Source: CAD feature listing. Evaluate the final solid. Frame: model axes, mm. A direction names the side the tool comes from. Give positions to 0.01 mm unless a question says otherwise; leave off trailing zeros. Order: outer loops, then holes, each group sorted by start corner. A loop starts at its lowest first (then second) coordinate and runs counter-clockwise, first axis right, second up. Notation, with made-up numbers: M -30,-6 L 3,-6 A17 cw 3,13 Z; hole C 3.5,-21 d6. An arc over 180 degrees is marked long. Use CSV: the item, a comma, the result in double quotes. Start each with the question number.
Item 1: Pull-direction query (Z, two-part tool) for faces 3 (the face through (57.719, 0.805, -94.535)), 4 (the face through (59.9, 0.8, -78.5)), 5 (the face through (59.97, 0.78, -120.62)), 6 (the face through (29.81, 0.78, -196.55)); classes: +Z half, -Z half, draft (parallel to the pull), parting line (faces both ways), or undercut.
Item 2: Section query A-A on z = -56.67. Return loops of the section in (x, y).
Item 3: First-contact query: pin 1 (0.5 mm diameter, centred on x = 16.5, y = 1, fed in from -Z); pin 2 (2.5 mm diameter, centred on x = 43.45, z = -42.87, fed in from -Y). Flat tips, straight axial feed; report the tip coordinate or a pass-through.
Item 4: Section query B-B on x = 55.5. Return loops of the section in (y, z), and give its area (3 significant figures).
Item 5: Access query for faces 1 (the face through (6.493, 0.783, -108.844)), 2 (the face through (3.66, 0.78, -167.99)). Directions: +Z, -Z, +X, -X, +Y, -Y. A direction counts if a zero-diameter tool reaches every point of the face in a straight line with its end or side. Return the directions, or none.
Item 6: Section query C-C on y = 0.3. Count the separate pieces of the cut face and the enclosed holes in it, and give its area (3 significant figures).
Item 7: Ray query, probe 1 along X at (y, z) = (0.8, -56.67); probe 2 along X at (y, z) = (0.25, -71); probe 3 along X at (y, z) = (0.65, -185). Return the intervals inside material, ascending. Write a range as from..to.
from build123d import *

# Parameters (mm, degrees)
SKETCH1_R           = 1.388229101
SKETCH1_R_2         = 1.896979128
SKETCH1_R_3         = 2
SKETCH1_R_4         = 1.314910669
SKETCH1_R_5         = 1.483383261
SKETCH1_R_6         = 1.248623853
SKETCH1_R_7         = 1.255629307
SKETCH1_R_8         = 7
SKETCH1_R_9         = 1.53911217
BOSS_EXTRUDE1_DEPTH = 1.5875
SKETCH4_W           = 66.272407177
SKETCH4_H           = 27.800260981
CUT_EXTRUDE2_DEPTH  = 20
FILLET3_R           = 10
FILLET4_R           = 10
BOSS_EXTRUDE3_START = -1.5875
BOSS_EXTRUDE3_DEPTH = 1.5875
SKETCH7_R           = 7
CUT_EXTRUDE3_DEPTH  = 1.5875
SKETCH8_W           = 100.106183873
SKETCH8_H           = 60.21728362
CUT_EXTRUDE4_DEPTH  = 35
FILLET5_R           = 10


with BuildPart() as part:
    # Sketch1 → Boss-Extrude1 (new body)
    with BuildSketch(Plane(origin=(0, 0, 0), x_dir=(1, 0, 0), z_dir=(0, 1, 0))):
        with BuildLine():
            Line((42.32729629, 228.6), (10.454309325, 228.6))
            Line((10.454309325, 228.6), (0, 135.362739137))
            Line((0, 135.362739137), (0, 0))
            Line((0, 0), (24.327009544, 0))
            Line((24.327009544, 0), (50.8, 0))
            Line((50.8, 0), (50.8, 64.87909603))
            Line((50.8, 64.87909603), (50.8, 87.423477361))
            Line((50.8, 87.423477361), (50.8, 98.200996728))
            ThreePointArc((50.8, 98.200996728), (50.4, 101.000996728), (50.8, 103.800996728))
            Line((50.8, 103.800996728), (50.8, 104.488200565))
            Line((50.8, 104.488200565), (50.8, 120.619222808))
            Line((50.8, 120.619222808), (50.8, 135.362739137))
            Line((50.8, 135.362739137), (42.32729629, 228.6))
        make_face()
        with Locations(Location((6.335590122, 44.288799513, 0), (0, 0, 270))):
            Circle(SKETCH1_R, mode=Mode.SUBTRACT)
        with Locations(Location((16.545548495, 56.66670766, 0), (0, 0, 270))):
            Circle(SKETCH1_R_2, mode=Mode.SUBTRACT)
        with Locations(Location((32.542900948, 56.67, 0), (0, 0, 270))):
            Circle(SKETCH1_R_3, mode=Mode.SUBTRACT)
        with Locations(Location((4.659546827, 82.793173401, 0), (0, 0, 270))):
            Circle(SKETCH1_R_4, mode=Mode.SUBTRACT)
        with Locations(Location((16.254490953, 72.66670766, 0), (0, 0, 270))):
            Circle(SKETCH1_R_3, mode=Mode.SUBTRACT)
        with Locations(Location((32.251843406, 72.67, 0), (0, 0, 270))):
            Circle(SKETCH1_R_3, mode=Mode.SUBTRACT)
        with BuildLine():
            Line((34.925740903, 92.78493524), (9.492033273, 92.78493524))
            ThreePointArc((9.492033273, 92.78493524), (6.992033273, 95.28493524), (9.492033273, 97.78493524))
            Line((9.492033273, 97.78493524), (34.925740903, 97.78493524))
            ThreePointArc((34.925740903, 97.78493524), (36.693507856, 97.052702193), (37.425740903, 95.28493524))
            ThreePointArc((37.425740903, 95.28493524), (36.693507856, 93.517168287), (34.925740903, 92.78493524))
        make_face(mode=Mode.SUBTRACT)
        with BuildLine():
            Line((34.925740903, 105.90993524), (9.492033273, 105.90993524))
            ThreePointArc((9.492033273, 105.90993524), (6.492033273, 108.90993524), (9.492033273, 111.90993524))
            Line((9.492033273, 111.90993524), (34.925740903, 111.90993524))
            ThreePointArc((34.925740903, 111.90993524), (37.047061246, 111.031255584), (37.925740903, 108.90993524))
            ThreePointArc((37.925740903, 108.90993524), (37.047061246, 106.788614896), (34.925740903, 105.90993524))
        make_face(mode=Mode.SUBTRACT)
        with Locations(Location((43.447673368, 42.868436544, 0), (0, 0, 270))):
            Circle(SKETCH1_R_5, mode=Mode.SUBTRACT)
        with Locations(Location((48.400988852, 71.551011715, 0), (0, 0, 270))):
            Circle(SKETCH1_R_6, mode=Mode.SUBTRACT)
        with Locations(Location((5.88467603, 135.103145298, 0), (0, 0, 270))):
            Circle(SKETCH1_R_7, mode=Mode.SUBTRACT)
        with BuildLine():
            Line((35.509675341, 119.784935244), (9.492033273, 119.784935244))
            ThreePointArc((9.492033273, 119.784935244), (7.026609419, 122.250359097), (9.492033273, 124.71578295))
            Line((9.492033273, 124.71578295), (35.509675341, 124.71578295))
            ThreePointArc((35.509675341, 124.71578295), (37.252993266, 123.993677022), (37.975099194, 122.250359097))
            ThreePointArc((37.975099194, 122.250359097), (37.252993266, 120.507041172), (35.509675341, 119.784935244))
        make_face(mode=Mode.SUBTRACT)
        with Locations(Location((29.504213454, 189.557234372, 0), (0, 0, 270))):
            Circle(SKETCH1_R_8, mode=Mode.SUBTRACT)
        with Locations(Location((45.747747887, 129.863467374, 0), (0, 0, 270))):
            Circle(SKETCH1_R_9, mode=Mode.SUBTRACT)
    extrude(amount=BOSS_EXTRUDE1_DEPTH)

    # Sketch4 → Cut-Extrude2 (cut)
    with BuildSketch(Plane(origin=(0, 0, -228.6), x_dir=(-1, 0, 0), z_dir=(0, 0, -1))):
        with Locations((-28.174690156, -1.980940155)):
            Rectangle(SKETCH4_W, SKETCH4_H)
    extrude(amount=-CUT_EXTRUDE2_DEPTH, mode=Mode.SUBTRACT)

    # Fillet3
    fillet3_edges = [part.edges().sort_by_distance(p)[0] for p in [
        (44.144746445, 0.79375, -208.6),
    ]]
    fillet(fillet3_edges, radius=FILLET3_R)

    # Fillet4
    fillet4_edges = [part.edges().sort_by_distance(p)[0] for p in [
        (50.8, 0.79375, 0),
        (0, 0.79375, 0),
        (8.211791854, 0.79375, -208.6),
    ]]
    fillet(fillet4_edges, radius=FILLET4_R)

    # Sketch6 → Boss-Extrude3 (add)
    with BuildSketch(Plane(origin=(0, 1.5875, 0), x_dir=(1, 0, 0), z_dir=(0, 1, 0)).offset(BOSS_EXTRUDE3_START)):
        with BuildLine():
            Line((50.8, 135.362739137), (50.8, 103.800996728))
            ThreePointArc((50.8, 103.800996728), (50.4, 101.000996728), (50.8, 98.200996728))
            Line((50.8, 98.200996728), (50.8, 61.124243317))
            Line((50.8, 61.124243317), (69.258211507, 96.360728536))
            ThreePointArc((69.258211507, 96.360728536), (70.393157133, 101.370875786), (68.890940865, 106.283413148))
            Line((68.890940865, 106.283413148), (50.8, 135.362739137))
        make_face()
    extrude(amount=BOSS_EXTRUDE3_DEPTH)

    # Sketch7 → Cut-Extrude3 (cut)
    with BuildSketch(Plane(origin=(0, 1.5875, 0), x_dir=(1, 0, 0), z_dir=(0, 1, 0))):
        with Locations(Location((60.4, 101.000996728, 0), (0, 0, 270))):
            Circle(SKETCH7_R)
    extrude(amount=-CUT_EXTRUDE3_DEPTH, mode=Mode.SUBTRACT)

    # Sketch8 → Cut-Extrude4 (cut)
    with BuildSketch(Plane.XY):
        with Locations((28.455154517, 1.704032249)):
            Rectangle(SKETCH8_W, SKETCH8_H)
    extrude(amount=-CUT_EXTRUDE4_DEPTH, mode=Mode.SUBTRACT)

    # Fillet5
    fillet5_edges = [part.edges().sort_by_distance(p)[0] for p in [
        (0, 0.79375, -35),
        (50.8, 0.79375, -35),
    ]]
    fillet(fillet5_edges, radius=FILLET5_R)


solid = part.part
Verdict:
1,face 3,"undercut"
1,face 4,"+Z half"
1,face 5,"-Z half"
1,face 6,"undercut"
2,outline,"M 0,0 L 14.65,0 L 14.65,1.59 L 0,1.59 Z; M 18.44,0 L 30.54,0 L 30.54,1.59 L 18.44,1.59 Z; M 34.54,0 L 50.8,0 L 50.8,1.59 L 34.54,1.59 Z"
3,pin 1,"z = -208.59"
3,pin 2,"through"
4,outline,"M 0,-127.81 L 1.59,-127.81 L 1.59,-106 L 0,-106 Z; M 0,-96 L 1.59,-96 L 1.59,-70.1 L 0,-70.1 Z"
4,area,"75.7 mm2"
5,face 1,"+Y, -Y"
5,face 2,"-Z, -X, +Y, -Y"
6,separate pieces,"1"
6,enclosed holes,"15"
6,area,"8,110 mm2"
7,probe 1,"0..14.65, 18.44..30.54, 34.54..50.8"
7,probe 2,"0..15.15, 17.36..31.15, 33.35..47.28, 49.52..55.97"
7,probe 3,"5.57..24.19, 34.82..46.29"
